from build123d import *

# Parameters (mm, degrees)
SKETCH1_W           = 12
SKETCH1_H           = 25
BOSS_EXTRUDE1_DEPTH = 2
BOSS_EXTRUDE2_DEPTH = 12
CUT_EXTRUDE1_REACH  = 20.446
SKETCH3_W           = 23.047029748
SKETCH3_H           = 41.13404119
SKETCH3_W_2         = 8
SKETCH3_H_2         = 35.39542334


with BuildPart() as part:
    # Sketch1 → Boss-Extrude1 (new body)
    with BuildSketch(Plane(origin=(0, 0, 0), x_dir=(0, 0, -1), z_dir=(1, 0, 0))):
        Rectangle(SKETCH1_W, SKETCH1_H)
    extrude(amount=BOSS_EXTRUDE1_DEPTH)

    # Sketch2 → Boss-Extrude2 (add)
    with BuildSketch(Plane.XY.offset(6)):
        with BuildLine():
            Line((-6, -9.5), (-6, -15.5))
            Line((-6, -15.5), (-5.4, -15.5))
            ThreePointArc((-5.4, -15.5), (-3.582605023, -12.411310958), (0, -12.5))
            Line((0, -12.5), (0, 2.5))
            ThreePointArc((0, 2.5), (-1.583592135, -4.208203932), (-6, -9.5))
        make_face()
    extrude(amount=-BOSS_EXTRUDE2_DEPTH)

    # Cut-Extrude1: up to this face of the body (flat: up to its plane)
    cut_extrude1_end = Plane(part.part.faces().sort_by_distance((0, 7.5, 0))[0])
    # Sketch3 → Cut-Extrude1 (cut, up to the picked face)
    with BuildSketch(Plane.ZY.offset(6), mode=Mode.PRIVATE) as cut_extrude1_sk1:
        Rectangle(SKETCH3_W, SKETCH3_H)
        Rectangle(SKETCH3_W_2, SKETCH3_H_2, mode=Mode.SUBTRACT)
    cut_extrude1_tool1 = split(extrude(cut_extrude1_sk1.sketch, amount=-CUT_EXTRUDE1_REACH, mode=Mode.PRIVATE), bisect_by=cut_extrude1_end, keep=Keep.BOTH, mode=Mode.PRIVATE)
    add(cut_extrude1_tool1.solids().sort_by(Axis((-6, 20.095515, 0), (1, 0, 0)))[0], mode=Mode.SUBTRACT)


solid = part.part
The listing builds one solid part. Answer for the finished solid, in the listing's coordinates (mm). A direction names the side the tool comes from. Round coordinates to 2 decimals unless told otherwise and drop trailing zeros. Write each loop counter-clockwise with the first axis right and the second up, starting at its lowest first coordinate (ties: lowest second). Pieces come first, ordered by that corner, then holes. Notation, with made-up numbers: M 25.5,-34.75 L 52.5,-34.75 A27 ccw 52.5,1.25 Z; hole C -26.75,-28 d8. An arc over 180 degrees is marked long. Write each question's results on one line, items separated by ' | '. Start each with the question number.
Item 1: Find section B-B on y = -5.25. Write down the section's boundary in (x, z), and give its area (3 significant figures).
Item 2: Find section A-A on z = -0.5. Write down the section's boundary in (x, y).
Item 3: Straight lines are drawn through the part: probe 1 along X at (y, z) = (-7, -4.5); probe 2 along Y at (x, z) = (0.25, -1.5); probe 3 along Z at (x, y) = (-0.25, -4.5). For each, find the intervals that lie inside material, in ascending order.
Item 4: Given pin 1 Ø1.5 at (y, z) = (-7.5, 4) entering from -X; pin 2 Ø2 at (x, z) = (1, -1.5) entering from -Y; pin 3 Ø6 at (y, z) = (-4, 2.5) entering from -X, each flat-ended and moving along its own axis, determine where each tip first touches the part or whether it passes through.
Item 5: Find section C-C on x = 1.5. Write down the section's boundary in (y, z).
Item 6: Which of the six approach directions +Z, -Z, +X, -X, +Y, -Y give full straight-line access (tool end or side, diameter ignored) to faces 1 (the cylindrical face through (-1.54, -4.12, 0.06)), 2 (the flat face through (1, -12.5, 0)), 3 (the flat face through (-3, -9, -4)), 4 (the flat face through (-3, -9, 4))?
Item 7: Find section D-D on y = 9. Write down the section's boundary in (x, z).
Item 8: The mould has two halves that part along X. Classify faces 5 (the flat face through (2, 0, 0)), 6 (the cylindrical face through (-3.63, -12.44, 0.06)), 7 (the flat face through (0, 3, 0)): +X half, -X half, draft (parallel to the pull), parting line (faces both ways), or undercut.
Answer block:
1) outline: M -2.16,-4 L 0,-4 L 0,-6 L 2,-6 L 2,6 L 0,6 L 0,4 L -2.16,4 Z | area: 41.3 mm²
2) outline: M -6,-15.5 L -5.4,-15.5 A3.53 cw 0,-12.5 L 2,-12.5 L 2,12.5 L 0,12.5 L 0,2.5 A15 cw -6,-9.5 Z
3) probe 1: x = 0 to 2 | probe 2: y = -12.5 to 12.5 | probe 3: z = -4 to 4
4) pin 1: stops at x = -4.54 | pin 2: stops at y = -12.5 | pin 3: stops at x = -3.39
5) outline: M -12.5,-6 L 12.5,-6 L 12.5,6 L -12.5,6 Z
6) face 1: +Z, -Z, -X, +Y | face 2: +Z, -Z, +X, -Y | face 3: -Z, -X, +Y, -Y | face 4: +Z, -X, +Y, -Y
7) outline: M 0,-6 L 2,-6 L 2,6 L 0,6 Z
8) face 5: +X half | face 6: undercut | face 7: -X half
